Verification items for the finished model (mm, model axes). Face numbers are marked on the shaded views. A direction names the side the tool comes from. Round coordinates to 2 decimals unless told otherwise and drop trailing zeros. Write each loop counter-clockwise with the first axis right and the second up, starting at its lowest first coordinate (ties: lowest second). Pieces come first, ordered by that corner, then holes. Notation, with made-up numbers: M 85,77 L 90,77 A30 cw 90,101 Z; hole C -8,62 d3. An arc over 180 degrees is marked long. One line per item, written item: value. Start each with the question number.
Item 1: Section check C-C, the plane x = 75. Record the cut outline in (y, z), then the cut area to 3 significant figures.
Item 2: Section check A-A, the plane z = 5.5. Record the cut outline in (x, y), then the cut area to 3 significant figures.
Item 3: Gauge pin test, flat ends, axial feed: pin 1 (2.5 mm diameter, centred on x = 43, y = 111, fed in from -Z); pin 2 (1.2 mm diameter, centred on x = 87, y = 111, fed in from +Z); pin 3 (2 mm diameter, centred on x = 77, y = 129.5, fed in from +Z); pin 4 (6 mm diameter, centred on x = 37.5, y = 102, fed in from +Z). Record the tip position at first contact, or that the pin passes through.
Item 4: Draft check along X on the marked faces 3, 4, 5 and 6. Enter one of: +X half, -X half, draft (parallel to the pull), parting line (faces both ways), or undercut.
Item 5: Thickness scan on probe 1 along X at (y, z) = (111, 0.45); probe 2 along Y at (x, z) = (43, 0.7); probe 3 along X at (y, z) = (24, 28). Record the ranges inside material, lowest first. Write a range as from..to.
Item 6: Section check B-B, the plane y = 52. Record the cut outline in (x, z), then the cut area to 3 significant figures.
Item 7: Tool access check on the marked faces 1 and 2. Record the directions out of +Z, -Z, +X, -X, +Y, -Y that give a thin tool (end or side, any length) a straight path to the whole face; none if there is none.
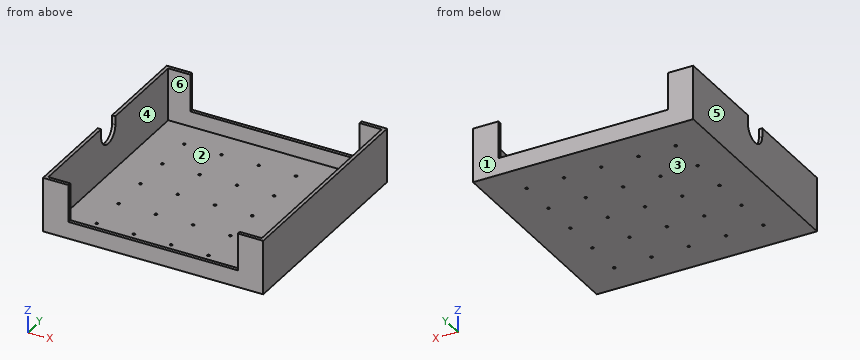
from build123d import *

# Parameters (mm, degrees)
ESQUISSE1_W             = 130
ESQUISSE1_H             = 130
BOSS_EXTRU_1_DEPTH      = 1
ESQUISSE2_W             = 130
ESQUISSE2_H             = 130
ESQUISSE2_W_2           = 126
ESQUISSE2_H_2           = 126
BOSS_EXTRU_2_DEPTH      = 31
ENL_V_MAT_EXTRU_1_DEPTH = 2
ESQUISSE6_W             = 100
ESQUISSE6_H             = 22
ENL_V_MAT_EXTRU_2_DEPTH = 187.611896727
ESQUISSE5_R             = 0.75
ENL_V_MAT_EXTRU_3_DEPTH = 1


with BuildPart() as part:
    # Esquisse1 → Boss.-Extru.1 (new body)
    with BuildSketch(Plane.XY):
        with Locations((65, 65)):
            Rectangle(ESQUISSE1_W, ESQUISSE1_H)
    extrude(amount=BOSS_EXTRU_1_DEPTH)

    # Esquisse2 → Boss.-Extru.2 (add)
    with BuildSketch(Plane.XY.offset(1)):
        with Locations((65, 65)):
            Rectangle(ESQUISSE2_W, ESQUISSE2_H)
        with Locations((65, 65)):
            Rectangle(ESQUISSE2_W_2, ESQUISSE2_H_2, mode=Mode.SUBTRACT)
    extrude(amount=BOSS_EXTRU_2_DEPTH)

    # Esquisse3 → Enlèv. mat.-Extru.1 (cut)
    with BuildSketch(Plane.ZY):
        with BuildLine():
            Line((32, 57.5), (32, 72.5))
            Line((32, 72.5), (27, 72.5))
            ThreePointArc((27, 72.5), (19.5, 65), (27, 57.5))
            Line((27, 57.5), (32, 57.5))
        make_face()
    extrude(amount=-ENL_V_MAT_EXTRU_1_DEPTH, mode=Mode.SUBTRACT)

    # Esquisse6 → Enlèv. mat.-Extru.2 (cut, through all)
    with BuildSketch(Plane(origin=(0, 130, 0), x_dir=(1, 0, 0), z_dir=(0, 1, 0))):
        with Locations((65, -21)):
            Rectangle(ESQUISSE6_W, ESQUISSE6_H)
    extrude(amount=-ENL_V_MAT_EXTRU_2_DEPTH, mode=Mode.SUBTRACT)

    # Esquisse5 → Enlèv. mat.-Extru.3 (cut)
    with BuildSketch(Plane(origin=(0, 0, 0), x_dir=(-1, 0, 0), z_dir=(0, 0, -1))):
        with Locations((-109, 111)):
            Circle(ESQUISSE5_R)
        with Locations((-87, 111)):
            Circle(ESQUISSE5_R)
        with Locations((-65, 111)):
            Circle(ESQUISSE5_R)
        with Locations((-43, 111)):
            Circle(ESQUISSE5_R)
        with Locations((-21, 111)):
            Circle(ESQUISSE5_R)
        with Locations((-109, 88)):
            Circle(ESQUISSE5_R)
        with Locations((-87, 88)):
            Circle(ESQUISSE5_R)
        with Locations((-65, 88)):
            Circle(ESQUISSE5_R)
        with Locations((-43, 88)):
            Circle(ESQUISSE5_R)
        with Locations((-21, 88)):
            Circle(ESQUISSE5_R)
        with Locations((-109, 65)):
            Circle(ESQUISSE5_R)
        with Locations((-87, 65)):
            Circle(ESQUISSE5_R)
        with Locations((-65, 65)):
            Circle(ESQUISSE5_R)
        with Locations((-43, 65)):
            Circle(ESQUISSE5_R)
        with Locations((-21, 65)):
            Circle(ESQUISSE5_R)
        with Locations((-109, 42)):
            Circle(ESQUISSE5_R)
        with Locations((-87, 42)):
            Circle(ESQUISSE5_R)
        with Locations((-65, 42)):
            Circle(ESQUISSE5_R)
        with Locations((-43, 42)):
            Circle(ESQUISSE5_R)
        with Locations((-21, 42)):
            Circle(ESQUISSE5_R)
        with Locations((-109, 19)):
            Circle(ESQUISSE5_R)
        with Locations((-87, 19)):
            Circle(ESQUISSE5_R)
        with Locations((-65, 19)):
            Circle(ESQUISSE5_R)
        with Locations((-43, 19)):
            Circle(ESQUISSE5_R)
        with Locations((-21, 19)):
            Circle(ESQUISSE5_R)
    extrude(amount=-ENL_V_MAT_EXTRU_3_DEPTH, mode=Mode.SUBTRACT)


solid = part.part
Response values:
1. outline: M 0,0 L 130,0 L 130,10 L 128,10 L 128,1 L 2,1 L 2,10 L 0,10 Z
1. area: 166 mm2
2. outline: M 0,0 L 130,0 L 130,130 L 0,130 Z; hole M 2,2 L 128,2 L 128,128 L 2,128 Z
2. area: 1,020 mm2
3. pin 1: stops at z = 0
3. pin 2: passes through
3. pin 3: stops at z = 10
3. pin 4: stops at z = 1
4. face 3: draft
4. face 4: undercut
4. face 5: -X half
4. face 6: undercut
5. probe 1: x = 0..20.25, 21.75..42.25, 43.75..64.25, 65.75..86.25, 87.75..108.25, 109.75..130
5. probe 2: y = 0..18.25, 19.75..41.25, 42.75..64.25, 65.75..87.25, 88.75..110.25, 111.75..130
5. probe 3: x = 0..2, 128..130
6. outline: M 0,0 L 130,0 L 130,32 L 128,32 L 128,1 L 2,1 L 2,32 L 0,32 Z
6. area: 254 mm2
7. face 1: +Z, -Z, +X, -X, +Y
7. face 2: +Z
